Model file for the job. Use its own axes, mm. A direction names the side the tool comes from. Coordinates: 2 decimals unless noted, no trailing zeros. Loops run counter-clockwise (first coordinate to the right, second up) from the corner with the lowest first, then second, coordinate; pieces in that order, holes last. Notation, with made-up numbers: M 51,32.5 L 73,32.5 A26 ccw 73,50.5 Z; hole C 65.25,37 d9. An arc over 180 degrees is marked long. One line per question, with ' | ' between items. Start each with the question number.
```python
from build123d import *

# Parameters (mm, degrees)
SKETCH1_R           = 80
SKETCH1_R_2         = 15
BOSS_EXTRUDE1_DEPTH = 65
CUT_EXTRUDE1_DEPTH  = 65
BOSS_EXTRUDE2_DEPTH = 65


with BuildPart() as part:
    # Sketch1 → Boss-Extrude1 (new body)
    with BuildSketch(Plane(origin=(0, 0, 0), x_dir=(0, 0, -1), z_dir=(1, 0, 0))):
        Circle(SKETCH1_R)
        Circle(SKETCH1_R_2, mode=Mode.SUBTRACT)
    extrude(amount=BOSS_EXTRUDE1_DEPTH)

    # Sketch2 → Cut-Extrude1 (cut)
    with BuildSketch(Plane(origin=(65, 0, 0), x_dir=(0, 0, -1), z_dir=(1, 0, 0))):
        with BuildLine():
            Line((-37.816442632, 49.5), (-61.776478803, 8))
            Line((-61.776478803, 8), (-22.627416998, 8))
            ThreePointArc((-22.627416998, 8), (-20.784609691, 12), (-18.241911729, 15.595917942))
            Line((-18.241911729, 15.595917942), (-37.816442632, 49.5))
        make_face()
        with BuildLine():
            Line((-61.776478803, -8), (-37.816442632, -49.5))
            Line((-37.816442632, -49.5), (-18.241911729, -15.595917942))
            ThreePointArc((-18.241911729, -15.595917942), (-20.784609691, -12), (-22.627416998, -8))
            Line((-22.627416998, -8), (-61.776478803, -8))
        make_face()
        with BuildLine():
            Line((-4.385505269, -23.595917942), (-23.960036171, -57.5))
            Line((-23.960036171, -57.5), (23.960036171, -57.5))
            Line((23.960036171, -57.5), (4.385505269, -23.595917942))
            ThreePointArc((4.385505269, -23.595917942), (0, -24), (-4.385505269, -23.595917942))
        make_face()
        with BuildLine():
            Line((18.241911729, -15.595917942), (37.816442632, -49.5))
            Line((37.816442632, -49.5), (61.776478803, -8))
            Line((61.776478803, -8), (22.627416998, -8))
            ThreePointArc((22.627416998, -8), (20.784609691, -12), (18.241911729, -15.595917942))
        make_face()
        with BuildLine():
            Line((22.627416998, 8), (61.776478803, 8))
            Line((61.776478803, 8), (37.816442632, 49.5))
            Line((37.816442632, 49.5), (18.241911729, 15.595917942))
            ThreePointArc((18.241911729, 15.595917942), (20.784609691, 12), (22.627416998, 8))
        make_face()
        with BuildLine():
            Line((23.960036171, 57.5), (-23.960036171, 57.5))
            Line((-23.960036171, 57.5), (-4.385505269, 23.595917942))
            ThreePointArc((-4.385505269, 23.595917942), (0, 24), (4.385505269, 23.595917942))
            Line((4.385505269, 23.595917942), (23.960036171, 57.5))
        make_face()
    extrude(amount=-CUT_EXTRUDE1_DEPTH, mode=Mode.SUBTRACT)

    # Sketch3 → Boss-Extrude2 (add)
    with BuildSketch(Plane(origin=(65, 0, 0), x_dir=(0, 0, -1), z_dir=(1, 0, 0))):
        Polygon((-5.254935121, 85.241193332), (4.745064879, 85.241193332), (3.011443405, 78.241193332), (-2.988556595, 78.241193332), align=None)
        Polygon((22.374626914, 75.034186847), (25.794612692, 81.383134846), (16.108781081, 83.870033718), (16.563127947, 76.52632617), align=None)
        Polygon((40.331930326, 67.112506447), (45.223390123, 72.411474692), (36.460323323, 77.229011433), (35.074090246, 70.003028491), align=None)
        Polygon((55.755030225, 54.973900443), (61.810615633, 58.889935272), (54.520929359, 65.735406331), (51.381218461, 59.081183079), align=None)
        Polygon((67.674836523, 39.381082095), (74.514052839, 41.668124637), (69.15578489, 50.111403892), (64.459875753, 44.447049648), align=None)
        Polygon((75.342383951, 21.313805526), (82.535498062, 21.828152487), (79.445328118, 31.338717649), (73.488281984, 27.020144624), align=None)
        Polygon((78.275892305, 1.907304169), (85.370934397, 0.616637237), (84.743029202, 10.596904521), (77.899149188, 7.895464539), align=None)
        Polygon((76.291038468, -17.619040124), (82.842200952, -20.633623598), (84.716014098, -10.810751091), (77.415326355, -11.72531662), align=None)
        Polygon((69.512538104, -36.038315328), (75.108187348, -40.587397978), (79.365980264, -31.539127453), (72.067213854, -30.609353013), align=None)
        Polygon((58.366309323, -52.19317064), (62.654850105, -57.990916872), (69.029090003, -50.285784444), (62.190853261, -47.570091183), align=None)
        Polygon((43.55271067, -65.068537087), (46.264678201, -71.750653184), (54.354848145, -65.872800661), (48.406812636, -61.541825573), align=None)
        Polygon((26.00253503, -73.855408044), (26.967526417, -81.002032075), (36.265291276, -77.320786548), (31.581193946, -71.646660728), align=None)
        Polygon((6.818524484, -78.001672092), (5.975905768, -85.163755387), (15.897052781, -83.910423051), (12.771212692, -77.249672691), align=None)
        Polygon((-12.793919032, -77.246804213), (-15.391203019, -83.974326737), (-5.470056006, -85.227659073), (-6.841230825, -77.998803615), align=None)
        Polygon((-31.602473563, -71.638235531), (-35.791225914, -77.508482303), (-26.493461056, -81.18972783), (-26.023814648, -73.846982847), align=None)
        Polygon((-48.425328454, -61.528373044), (-53.942354455, -66.172494869), (-45.852184511, -72.050347392), (-43.571226488, -65.055084558), align=None)
        Polygon((-62.205441863, -47.552456593), (-68.704086479, -50.678646217), (-62.329846582, -58.383778645), (-58.380897924, -52.175536049), align=None)
        Polygon((-72.076958583, -30.588644408), (-79.148888074, -32.00047184), (-74.891095158, -41.048742365), (-69.522282834, -36.017606723), align=None)
        Polygon((-77.419614916, -11.702835198), (-84.620473942, -11.311590128), (-82.746660796, -21.134462636), (-76.295327028, -17.596558703), align=None)
        Polygon((-77.897712113, 7.918306187), (-84.775044219, 10.088040392), (-85.402949415, 0.107773108), (-78.27445523, 1.930145817), align=None)
        Polygon((-73.481209571, 27.041911273), (-79.602886688, 30.853802234), (-82.693056632, 21.343237071), (-75.335311537, 21.335572176), align=None)
        Polygon((-64.447612387, 44.466373621), (-69.428987027, 49.680906209), (-74.787254977, 41.237626954), (-67.662573157, 39.400406068), align=None)
        Polygon((-51.364534694, 59.096850178), (-54.892608769, 65.386376133), (-62.182295043, 58.540905074), (-55.738346459, 54.989567543), align=None)
        Polygon((-35.054034381, 70.014054296), (-36.907126021, 76.983379571), (-45.670192822, 72.16584283), (-40.311874462, 67.123532251), align=None)
        Polygon((-16.540960169, 76.532017888), (-16.602632811, 83.743234145), (-26.288464422, 81.256335273), (-22.352459135, 75.039878565), align=None)
    extrude(amount=-BOSS_EXTRUDE2_DEPTH)


solid = part.part
```
(1) Two-plate mould, pull along Z, no slides. Class faces 5 (the face through (32.96, 26.52, -81.01)), 6 (the face through (32.955, -84.592, 10.5)), 7 (the face through (32.955, -12.053, 20.754)): pulls with the +Z half, pulls with the -Z half, needs draft (parallel to the pull), parting line crosses it, or undercut.
(2) Band-saw the part on B-B on x = 6.5. Give the number of separate pieces and of enclosed holes in the cut face, then the cut area to 3 significant figures.
(3) Drill centre lines: line 1 (Y direction, x = 27.5, z = 0); line 2 (Z direction, x = 16, y = -23); line 3 (Y direction, x = 51, z = -33.5). Where is each one in solid material? Low to high. Write a range as [from, to].
(4) 3-axis set-ups, long thin cutter, end or side, ignore diameter. For faces 1 (the face through (32.96, 32.79, -28.17)), 2 (the face through (32.955, 40.788, -71.881)), 3 (the face through (32.955, -39.164, 72.88)), 4 (the face through (32.955, 82.517, 21.378)): which of +Z, -Z, +X, -X, +Y, -Y reach the whole face in a straight line?
(5) Pin check, flat tips, straight feed: P1, Ø1, axis at y = -13.5, z = -21.5, coming from the +X side (1 decimal); P2, Ø6, axis at x = 22, y = -3.5, coming from the -Z side; P3, Ø11.5, axis at x = 46, z = 36.5, coming from the -Y side; P4, Ø5, axis at x = 9.5, y = -27, coming from the -Z side. Stop position of each tip, or through.
(6) Band-saw the part on A-A on z = 0. Write the cut outline in (x, y), then the cut area to 3 significant figures.
Computed values:
1) face 5: pulls with the -Z half | face 6: pulls with the +Z half | face 7: undercut
2) separate pieces: 1 | enclosed holes: 7 | area: 14,800 mm^2
3) line 1: [-80, -57.5], [-24, -15], [15, 24], [57.5, 85.24] | line 2: [-76.62, -53.12], [-22.52, 22.52], [53.12, 76.62] | line 3: [-78.42, -73.97], [-72.65, -42.02], [-8, 8], [42.02, 72.65]
4) face 1: +X, -X | face 2: -Z, +X, -X | face 3: +X, -X, -Y | face 4: +Z, +X, -X, +Y
5) P1: through | P2: z = -80 | P3: y = -79.5 | P4: z = -76.16
6) outline: M 0,-80 L 65,-80 L 65,-57.5 L 0,-57.5 Z; M 0,-24 L 65,-24 L 65,-15 L 0,-15 Z; M 0,15 L 65,15 L 65,24 L 0,24 Z; M 0,57.5 L 65,57.5 L 65,85.24 L 0,85.24 Z | area: 4,440 mm^2
